Could you check a few things on this drawing? It's one solid part, dimensions in mm from its lowest x, y, z. Round coordinates to 2 decimals unless told otherwise and drop trailing zeros. Loops run counter-clockwise (first coordinate to the right, second up) from the corner with the lowest first, then second, coordinate; pieces in that order, holes last. Notation, with made-up numbers: (77, 47.5) -> (122, 47.5) arc R25 cw to (122, 79.5) -> close; hole circle Ø11 at (6, -26.5). An arc over 180 degrees is marked (long way). Use one line per item in the form item = value. Start each with the question number.
Item 1: If we section it at A-A (x = 13): Write out the boundary of the cut face in (y, z).
Item 2: Thinking about a two-plate mould opening in Y: for the marked faces 1, 2 and 3, which applies, released by +Y, released by -Y, zero draft, split by the parting line, or undercut?
Item 3: I'm going to push flat-ended pins straight in: pin 1 Ø3 at (x, z) = (14, 5.5) entering from -Y; pin 2 Ø1 at (x, y) = (22, 23) entering from -Z; pin 3 Ø1 at (y, z) = (10, 8) entering from +X; pin 4 Ø1.5 at (y, z) = (20.5, 9.5) entering from +X. Where does each tip first touch, or does it pass through?
Item 4: If I drill on L1, parallel to Y at x = 13, z = 7; L2, parallel to Y at x = 8, z = 4; L3, parallel to X at y = 11, z = 7, over which ranges is the centre line in solid material (lowest first)? Write a range as [from, to].
Item 5: If we section it at C-C (z = 16.25): Write out the boundary of the cut face in (x, y), then the cut area to 3 significant figures.
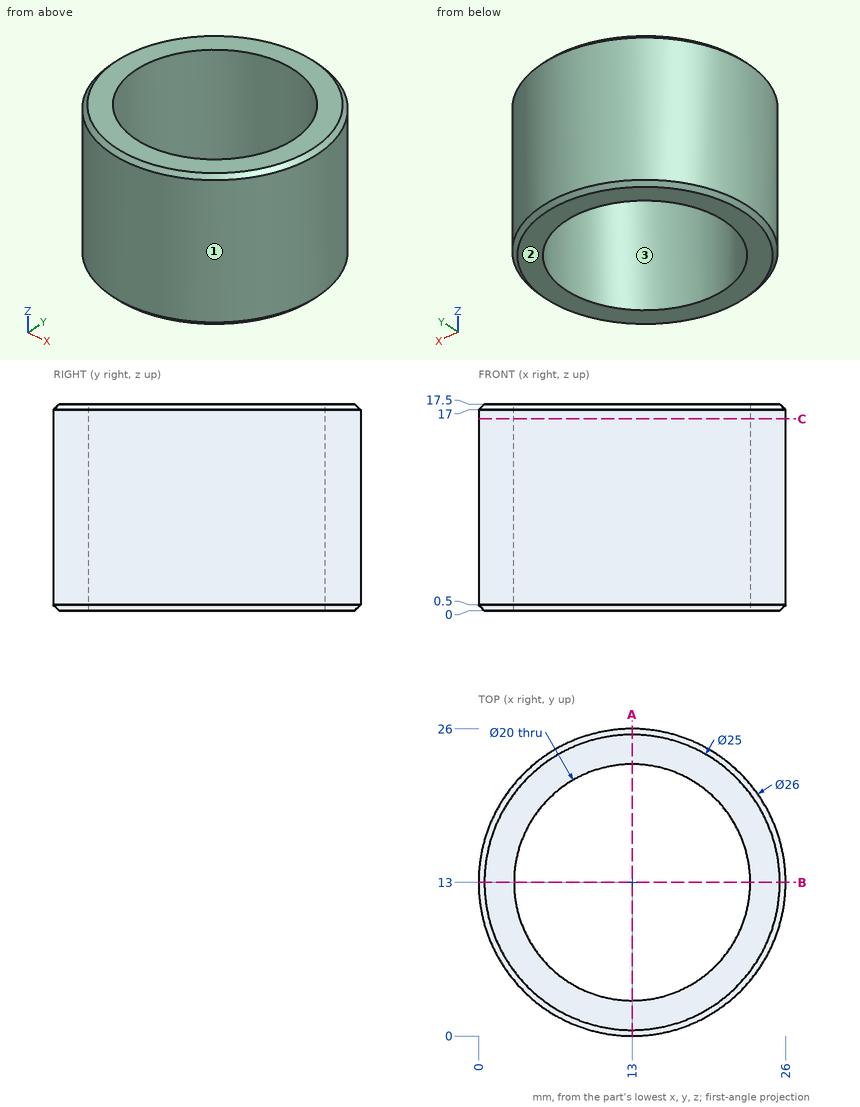
Values found:
q1.outline = (0, 0.5) -> (0.5, 0) -> (3, 0) -> (3, 17.5) -> (0.5, 17.5) -> (0, 17) -> close; (23, 0) -> (25.5, 0) -> (26, 0.5) -> (26, 17) -> (25.5, 17.5) -> (23, 17.5) -> close
q2.face_1 = split by the parting line
q2.face_2 = zero draft
q2.face_3 = undercut
q3.pin_1 = 0
q3.pin_2 = 0.45
q3.pin_3 = 25.76
q3.pin_4 = 24.11
q4.L1 = [0, 3], [23, 26]
q4.L2 = [1, 4.34], [21.66, 25]
q4.L3 = [0.15, 3.2], [22.8, 25.85]
q5.outline = circle Ø26 at (13, 13); hole circle Ø20 at (13, 13)
q5.area = 217 mm2
